Read the model definition and answer for the solid it produces. Units are mm, in the model's axes. Give positions to 0.01 mm unless a question says otherwise; leave off trailing zeros. Loops run counter-clockwise (first coordinate to the right, second up) from the corner with the lowest first, then second, coordinate; pieces in that order, holes last. Notation, with made-up numbers: (79.25, 23.5) - (116.25, 23.5) arc R26 cw to (116.25, 40.5) - close; hole circle Ø2 at (49.5, 87.25). An arc over 180 degrees is marked (long way). Write item = value, one per line.
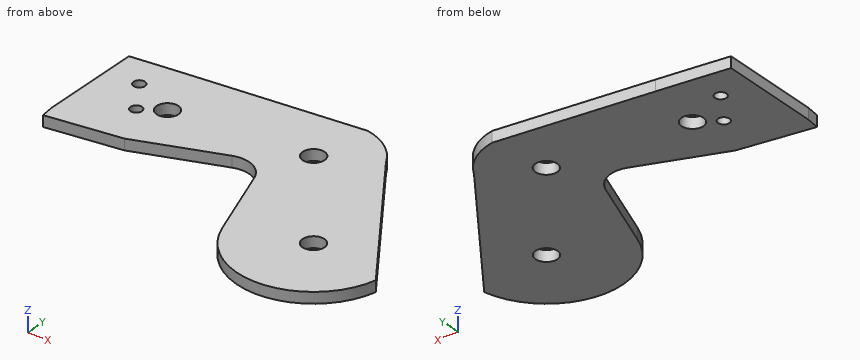
```python
from build123d import *

# Parameters (mm, degrees)
SKETCH_1_R      = 4
SKETCH_1_R_2    = 2.1
EXTRUDE_1_DEPTH = 4


with BuildPart() as part:
    # 草图1 → 凸台-拉伸1 (new body)
    with BuildSketch(Plane.XY):
        with BuildLine():
            Line((27.595444366, 44.436718371), (58.424396384, 55.525816351))
            ThreePointArc((58.424396384, 55.525816351), (66.108542504, 55.144576239), (71.247769486, 49.419212353))
            Line((71.247769486, 49.419212353), (81.175756204, 21.050380059))
            ThreePointArc((81.175756204, 21.050380059), (109.210938469, 2.084714208), (134.977054883, 24.034091663))
            Line((134.977054883, 24.034091663), (96.380255963, 79.649048221))
            ThreePointArc((96.380255963, 79.649048221), (90.097204959, 87.005823858), (81.213704463, 90.837572367))
            Line((81.213704463, 90.837572367), (25.665757334, 85.467931148))
            ThreePointArc((25.665757334, 85.467931148), (12.828050908, 84.180051983), (0, 82.799309813))
            Line((0, 82.799309813), (0, 45.6506733))
            Line((0, 45.6506733), (0.554484915, 40.773047428))
            Line((0.554484915, 40.773047428), (27.595444366, 44.436718371))
        make_face()
        with Locations((27.644326344, 65)):
            Circle(SKETCH_1_R, mode=Mode.SUBTRACT)
        with Locations((107.662812973, 30)):
            Circle(SKETCH_1_R, mode=Mode.SUBTRACT)
        with Locations((77.412339268, 69.810913587)):
            Circle(SKETCH_1_R, mode=Mode.SUBTRACT)
        with Locations((20, 60)):
            Circle(SKETCH_1_R_2, mode=Mode.SUBTRACT)
        with Locations((12, 72)):
            Circle(SKETCH_1_R_2, mode=Mode.SUBTRACT)
    extrude(amount=EXTRUDE_1_DEPTH)


solid = part.part
```
1) Each of these flat-tipped pins is pushed along its axis until it touches: P1, Ø6.5, axis at x = 20, y = 60, coming from the -Z side; P2, Ø1, axis at x = 33.5, z = 1, coming from the -Y side; P3, Ø1.5, axis at x = 88.5, z = 3.5, coming from the -Y side; P4, Ø1, axis at x = 58.5, z = 1.5, coming from the -Y side. Where does it stop, or does it pass through?
Output:
P1 = 0
P2 = 46.38
P3 = 8.96
P4 = 55.37
2) A cutting plane is placed at B-B on x = 12. Determine the outline of the cut face in (y, z).
Output:
outline = (42.32, 0) - (69.9, 0) - (69.9, 4) - (42.32, 4) - close; (74.1, 0) - (84.09, 0) - (84.09, 4) - (74.1, 4) - close
3) A cutting plane is placed at A-A on y = 72. Determine the outline of the cut face in (x, z).
Output:
outline = (0, 0) - (9.9, 0) - (9.9, 4) - (0, 4) - close; (14.1, 0) - (74.06, 0) - (74.06, 4) - (14.1, 4) - close; (80.76, 0) - (101.69, 0) - (101.69, 4) - (80.76, 4) - close
4) Find the intervals of material crossed by probe 1 along X at (y, z) = (71, 3); probe 2 along X at (y, z) = (28, 1.6); probe 3 along Y at (x, z) = (26, 3.5), in increasing order.
Output:
probe_1 = 0 to 10.15, 13.85 to 73.59, 81.23 to 102.38
probe_2 = 78.74 to 104.2, 111.13 to 132.22
probe_3 = 44.22 to 61.35, 68.65 to 85.5
5) A cutting plane is placed at D-D on z = 1.3. Determine the outline of the cut face in (x, y), then the cut area to 3 significant figures.
Output:
outline = (0, 45.65) - (0.55, 40.77) - (27.6, 44.44) - (58.42, 55.53) arc R10 cw to (71.25, 49.42) - (81.18, 21.05) arc R27.96 ccw to (134.98, 24.03) - (96.38, 79.65) arc R21.37 ccw to (81.21, 90.84) - (25.67, 85.47) arc R1782.98 ccw to (0, 82.8) - close; hole circle Ø4.2 at (12, 72); hole circle Ø4.2 at (20, 60); hole circle Ø8 at (27.64, 65); hole circle Ø8 at (77.41, 69.81); hole circle Ø8 at (107.66, 30)
area = 6,030 mm²
6) A cutting plane is placed at C-C on y = 30. Determine the outline of the cut face in (x, z).
Output:
outline = (78.04, 0) - (103.66, 0) - (103.66, 4) - (78.04, 4) - close; (111.66, 0) - (130.84, 0) - (130.84, 4) - (111.66, 4) - close
